Autodesk Inventor part; units mm, degrees
ref_plane "YZ Plane" through (0, 0, 0) normal (1, 0, 0) x (0, 1, 0)
ref_plane "XZ Plane" through (0, 0, 0) normal (0, 1, 0) x (-1, 0, 0)
ref_plane "XY Plane" through (0, 0, 0) normal (0, 0, 1) x (1, 0, 0)
sketch "Sketch_40" plane through (0, 0, 0) normal (0, 0, 1) x (1, 0, 0)
  line L0 (2.5, 0) -> (-2.5, 0)
  line L1 (0, 6.295) -> (0, 5.3)
  arc A0 (0, 5.3) -> (0.3, 5) centre (0.3, 5.3) ccw
  line L2 (0.3, 5) -> (4.7, 5)
  arc A1 (4.7, 5) -> (5, 5.3) centre (4.7, 5.3) ccw
  line L3 (5, 5.3) -> (5, 6.295)
  arc A2 (5, 6.295) -> (4.925, 6.37) centre (4.925, 6.295) ccw
  line L4 (4.925, 6.37) -> (3.3018, 6.37)
  arc A3 (1.6982, 6.37) -> (3.3018, 6.37) centre (2.5, 7.25) ccw
  line L5 (1.6982, 6.37) -> (0.075, 6.37)
  arc A4 (0.075, 6.37) -> (0, 6.295) centre (0.075, 6.295) ccw
revolve "Revolution1" add sketch "Sketch_40" angle 360 about axis through (2.5, 0, 0) along (1, 0, 0)
sketch "Sketch_42" plane through (0, 0, 0) normal (0, 0, 1) x (1, 0, 0)
  line L0 (2.5, 0) -> (-2.5, 0)
  line L1 (0, 13.15) -> (0, 5.9)
  line L2 (0, 5.9) -> (0.15, 5.9)
  arc A0 (0.15, 5.9) -> (0.45, 6.2) centre (0.15, 6.2) ccw
  line L3 (0.45, 6.2) -> (0.45, 12.85)
  line L4 (0.45, 12.85) -> (4.55, 12.85)
  line L5 (4.55, 12.85) -> (4.55, 6.2)
  arc A1 (4.55, 6.2) -> (4.85, 5.9) centre (4.85, 6.2) ccw
  line L6 (4.85, 5.9) -> (5, 5.9)
  line L7 (5, 5.9) -> (5, 13.15)
  line L8 (5, 13.15) -> (0, 13.15)
revolve "Revolution2" cut sketch "Sketch_42" angle 360 about axis through (2.5, 0, 0) along (1, 0, 0)
sketch "Sketch_44" plane through (0, 0, 0) normal (0, 0, 1) x (1, 0, 0)
  line L0 (5, 0) -> (-5, 0)
  line L1 (4.745, 6.4513) -> (4.835, 5.9)
  line L2 (4.835, 5.9) -> (4.925, 5.9)
  line L3 (4.925, 5.9) -> (4.88, 6.4513)
  line L4 (4.88, 6.4513) -> (4.925, 7.0025)
  line L5 (4.925, 7.0025) -> (4.925, 8.575)
  line L6 (4.925, 8.575) -> (4.8734, 8.575)
  line L7 (4.8734, 8.575) -> (4.745, 7.0025)
  line L8 (4.745, 7.0025) -> (4.745, 6.4513)
revolve "Revolution3" add sketch "Sketch_44" angle 360 about axis through (5, 0, 0) along (1, 0, 0)
sketch "Sketch_49" plane through (0, 0, 0) normal (0, 0, 1) x (1, 0, 0)
  line L0 (5, 0) -> (-5, 0)
  line L1 (0.105, 5.9) -> (0.195, 5.9)
  line L2 (0.195, 5.9) -> (0.285, 6.4513)
  line L3 (0.285, 6.4513) -> (0.285, 7.0025)
  line L4 (0.285, 7.0025) -> (0.1566, 8.575)
  line L5 (0.1566, 8.575) -> (0.105, 8.575)
  line L6 (0.105, 8.575) -> (0.105, 7.0025)
  line L7 (0.105, 7.0025) -> (0.15, 6.4513)
  line L8 (0.15, 6.4513) -> (0.105, 5.9)
revolve "Revolution4" add sketch "Sketch_49" angle 360 about axis through (5, 0, 0) along (1, 0, 0)
properties part number "SKF_W 61800 R-2RS1_PART1"
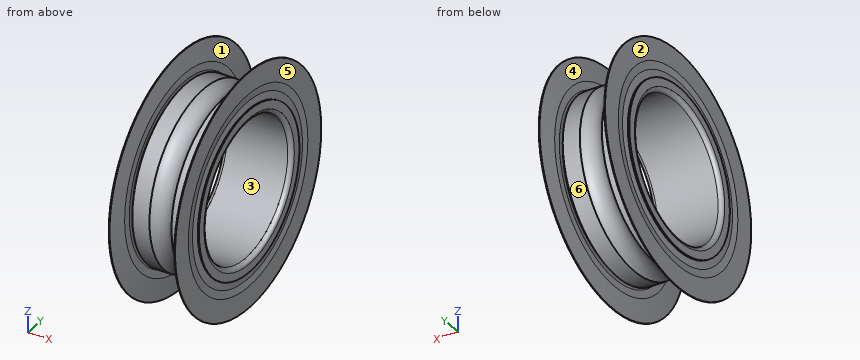
Verification items for the finished model (mm, model axes). Face numbers are marked on the shaded views. A direction names the side the tool comes from. Give positions to 0.01 mm unless a question says otherwise; leave off trailing zeros. Order: outer loops, then holes, each group sorted by start corner. A loop starts at its lowest first (then second) coordinate and runs counter-clockwise, first axis right, second up. Notation, with made-up numbers: M 38,0.25 L 62,0.25 A20 cw 62,17.25 Z; hole C 83.25,36.25 d8. An arc over 180 degrees is marked long. Answer in a Markdown table with one row per item. Add a question column.
Item 1: Section check A-A, the plane x = 3.7. Enter the section's corners in (y, z), and give its area (3 significant figures).
Item 2: Scan lines: probe 1 along Z at (x, y) = (1.25, 0); probe 2 along Z at (x, y) = (3, -1.5); probe 3 along Y at (x, z) = (4.6, 1.25). Record each from-to range of solid material in increasing order. Write a range as from..to.
Item 3: Mould release check, pull along X, two halves, no side actions. Record for the marked faces 1, 2, 3 and 4: released by +X, released by -X, zero draft, split by the parting line, or undercut.
Item 4: Gauge pin test, flat ends, axial feed: pin 1 (10 mm diameter, centred on y = 0.5, z = -2, fed in from +X); pin 2 (2 mm diameter, centred on x = 3.5, y = 2, fed in from +Z); pin 3 (1 mm diameter, centred on x = 2, z = -4.5, fed in from +Y); pin 4 (1.5 mm diameter, centred on x = 2.5, z = -3.5, fed in from -Y). Record the tip position at first contact, or that the pin passes through.
Item 5: Tool access check on the marked faces 5 and 6. Record the directions out of +Z, -Z, +X, -X, +Y, -Y that give a thin tool (end or side, any length) a straight path to the whole face; none if there is none.
Filled sheet:
| question | item | result |
|---|---|---|
| 1 | outline | C 0,0 d12.74; hole C 0,0 d10 |
| 1 | area | 48.9 mm^2 |
| 2 | probe 1 | z = -6.37..-5, 5..6.37 |
| 2 | probe 2 | z = -5.98..-4.77, 4.77..5.98 |
| 2 | probe 3 | y = -5.9..-4.84, 4.84..5.9 |
| 3 | face 1 | undercut |
| 3 | face 2 | released by -X |
| 3 | face 3 | zero draft |
| 3 | face 4 | undercut |
| 4 | pin 1 | stops at x = 5 |
| 4 | pin 2 | stops at z = 6.29 |
| 4 | pin 3 | stops at y = 4.87 |
| 4 | pin 4 | stops at y = -5.42 |
| 5 | face 5 | +X |
| 5 | face 6 | none |
